Autodesk Inventor part; units mm, degrees
ref_plane "Work Plane3" through (25.4, 13.0175, 0) normal (1, 0, 0) x (0, 0, -1)
ref_plane "YZ Plane" through (0, 0, 0) normal (1, 0, 0) x (0, 1, 0)
ref_plane "XZ Plane" through (0, 0, 0) normal (0, 1, 0) x (-1, 0, 0)
sketch "Sketch1" plane through (0, 0, 0) normal (0, 1, 0) x (-1, 0, 0)
  line L0 (0, 0) -> (-50.8, 0)
  line L1 (-50.8, 0) -> (-50.8, -25.4)
  line L2 (-50.8, -25.4) -> (0, -25.4)
  line L3 (0, -25.4) -> (0, 0)
  dimension "d0" = 50.8
  dimension "d1" = 25.4
extrude "Extrusion1" add sketch "Sketch1" along normal blind 3.175
sketch "Sketch10" plane through (0, 3.175, 0) normal (0, 1, 0) x (1, 0, 0)
  line L0 (50.8, 25.4) -> (0, 25.4)
  line L1 (0, 25.4) -> (50.8, 25.4)
  line L2 (50.8, 25.4) -> (50.8, 31.75)
  line L3 (50.8, 31.75) -> (0, 31.75)
  line L4 (0, 31.75) -> (0, 25.4)
  point P0 (0, 0)
  dimension "d46" = 6.35
extrude "Extrusion7" add sketch "Sketch10" against normal blind 57.15
sketch "Sketch11" plane through (50.8, 0, 0) normal (1, 0, 0) x (0, 0, -1)
  line L0 (25.4, -53.975) -> (31.75, -53.975)
  line L1 (25.4, -53.975) -> (0, -53.975)
  line L2 (0, -53.975) -> (0, -50.8)
  line L3 (0, -50.8) -> (25.4, -50.8)
  line L4 (25.4, -50.8) -> (25.4, -53.975)
  point P0 (0, 0)
  dimension "d49" = 3.175
  dimension "d80" = 25.4
extrude "Extrusion8" add sketch "Sketch11" against normal blind 50.8
sketch "Sketch12" plane through (0, 3.175, 0) normal (0, 1, 0) x (1, 0, 0)
  line L0 (9.525, 31.75) -> (19.05, 31.75)
  line L1 (19.05, 31.75) -> (19.05, 0)
  line L2 (19.05, 0) -> (9.525, 0)
  line L3 (9.525, 0) -> (9.525, 31.75)
  line L4 (31.75, 31.75) -> (41.275, 31.75)
  line L5 (41.275, 31.75) -> (41.275, 0)
  line L6 (41.275, 0) -> (31.75, 0)
  line L7 (31.75, 0) -> (31.75, 31.75)
  line L8 (19.05, 31.75) -> (31.75, 31.75) construction
  line L9 (50.8, 25.4) -> (0, 25.4) construction
  line L10 (50.8, 31.75) -> (0, 31.75) construction
  line L11 (50.8, 0) -> (50.8, 31.75) construction
  point P0 (0, 0)
  point P1 (25.4, 31.75)
  point P2 (25.4, 31.75)
  point P3 (41.275, 15.875)
  point P4 (50.8, 15.875)
  point P5 (36.5125, 31.75)
  point P6 (25.4, 31.75)
  dimension "d52" = 12.7
  dimension "d54" = 9.525
extrude "Extrusion9" add sketch "Sketch12" along normal blind 76.2
sketch "Sketch14" plane through (0, 3.175, 0) normal (0, 1, 0) x (1, 0, 0)
  line L0 (0, 31.75) -> (0, 0)
  line L1 (0, 0) -> (50.8, 0)
  point P0 (12.7, 12.7)
  point P1 (38.1, 12.7)
  dimension "d62" = 12.7
  dimension "d63" = 12.7
  dimension "d64" = 25.4
hole "Hole3" at (12.7, 3.175, -12.7) at (38.1, 3.175, -12.7) direction (0, -1, 0) diameter 3.175 end through all
sketch "Sketch15" plane through (50.8, 3.175, -31.75) normal (0, 0, -1) x (-1, 0, 0)
  line L0 (6.35, -9.525) -> (44.45, -9.525) construction
  line L1 (44.45, -9.525) -> (44.45, -47.625) construction
  line L2 (44.45, -47.625) -> (6.35, -47.625) construction
  line L3 (6.35, -47.625) -> (6.35, -9.525) construction
  line L4 (0, 0) -> (50.8, 0) construction
  line L5 (50.8, 0) -> (50.8, -57.15) construction
  point P0 (50.8, -3.175)
  point P1 (25.4, -9.525)
  point P2 (25.4, 0)
  point P3 (44.45, -28.575)
  point P4 (50.8, -28.575)
  dimension "d72" = 38.1
hole "Hole4" at (44.45, -6.35, -31.75) at (6.35, -6.35, -31.75) at (6.35, -44.45, -31.75) at (44.45, -44.45, -31.75) direction (0, 0, 1) diameter 3.175 end through all
sketch "Sketch17" plane through (9.525, 3.175, -31.75) normal (-1, 0, 0) x (0, 0, 1)
  circle A0 centre (14.2875, 31.75) radius 14.2875
  line L0 (0, 0) -> (31.75, 0)
  line L1 (31.75, 0) -> (31.75, 76.2)
  line L2 (0, 76.2) -> (31.75, 76.2)
  line L3 (31.75, 76.2) -> (0, 76.2)
  line L4 (0, 76.2) -> (0, 33.9421)
  line L5 (0, 0) -> (0, 76.2)
  arc A1 (31.75, 42.7485) -> (0, 46.6421) centre (14.2875, 31.75) ccw
  arc A2 (0, 46.6421) -> (0, 0) centre (22.3743, 23.321) ccw
  point P0 (31.75, -3.175)
  point P1 (31.75, 30.0485)
  point P2 (0, 46.6421)
  point P3 (0, 46.6421)
  point P4 (0, 46.6421)
  dimension "d83" = 28.575
  dimension "d84" = 31.75
  dimension "d85" = 17.4625
  dimension "d98" = 6.35
extrude "Extrusion16" cut sketch "Sketch17" against normal blind 38.1 contours A0 | L4 L2 L1 A1
sketch "Sketch19" plane through (0, 0, 0) normal (0, 0, 1) x (1, 0, 0)
  line L0 (31.75, 3.175) -> (31.75, 20.0329)
  arc A0 (19.05, 15.875) -> (31.75, 15.875) centre (25.4, 14.4462) ccw
  line L1 (19.05, 3.175) -> (31.75, 3.175)
  line L2 (19.05, 3.175) -> (19.05, 45.9235)
  line L3 (31.75, 3.175) -> (31.75, 45.9235)
  point P0 (0, 0)
  point P1 (31.75, 15.875)
  dimension "d103" = 4.7625
  dimension "d104" = 12.7
  dimension "d105" = 12.7
extrude "Extrusion18" add sketch "Sketch19" against normal blind 31.75
sketch "Sketch20" plane through (19.05, 34.925, -17.4625) normal (1, 0, 0) x (0, 0, -1)
  circle A0 centre (0, 0) radius 14.2875
  circle A1 centre (0, 0) radius 15.5575
  point P0 (-17.4625, -34.925)
  dimension "d108" = 1.27
extrude "Extrusion20" add sketch "Sketch17" against normal blind 9.525 contours L5 A2 L4
extrude "Extrusion21" cut sketch "Sketch20" against normal blind 1.651
ref_plane "Work Plane3" through (25.4, 13.0175, 0) normal (1, 0, 0) x (0, 0, -1)
mirror "Mirror6" about plane through (25.4, 13.0175, 0) normal (1, 0, 0) of "Extrusion20", "Extrusion21"
sketch "Sketch21" plane through (41.275, 3.175, 0) normal (1, 0, 0) x (0, 0, -1)
  circle A0 centre (17.4625, 31.75) radius 14.2875
  arc A1 (31.75, 0) -> (31.75, 46.6421) centre (9.3757, 23.321) ccw
  arc A2 (31.75, 46.6421) -> (0, 42.7485) centre (17.4625, 31.75) ccw
  line L0 (0, 0) -> (0, 42.7485)
  line L1 (31.75, 0) -> (0, 0)
  point P0 (0, -3.175)
sketch "Sketch22" plane through (0, 3.175, 0) normal (0, 1, 0) x (1, 0, 0)
  line L0 (50.8, 0) -> (50.8, 31.75)
  line L1 (41.275, 31.75) -> (41.275, 0)
  line L2 (41.275, 0) -> (50.8, 0)
  line L3 (50.8, 0) -> (50.8, 31.75)
  line L4 (50.8, 31.75) -> (41.275, 31.75)
  point P0 (0, 0)
sketch "Sketch23" plane through (41.275, 3.175, 0) normal (1, 0, 0) x (0, 0, -1)
  circle A0 centre (17.4625, 31.75) radius 14.2875
  line L0 (14.1389, 17.8544) -> (0, 17.8544)
  line L1 (0, 0) -> (0, 42.7485)
  line L2 (14.1389, 17.8544) -> (31.75, 17.8544)
  line L3 (31.75, 0) -> (31.75, 9.8425)
  line L4 (31.75, 17.8544) -> (31.75, 0)
  point P0 (0, -3.175)
sketch "Sketch24" plane through (0, 0, 0) normal (0, 0, 1) x (1, 0, 0)
  line L0 (50.8, 0) -> (50.8, 3.175)
  line L1 (50.8, 3.175) -> (41.275, 19.9074)
  line L2 (41.275, 49.8171) -> (41.275, 3.175)
  line L3 (41.275, 21.0294) -> (41.275, 3.175)
  line L4 (41.275, 3.175) -> (50.8, 3.175)
  line L5 (41.275, 3.175) -> (50.8, 3.175)
  point P0 (0, 0)
extrude "Extrusion22" add sketch "Sketch24" against normal blind 31.75
mirror "Mirror7" about plane through (25.4, 13.0175, 0) normal (1, 0, 0) of "Extrusion22"
properties part number "Intake - Mount"
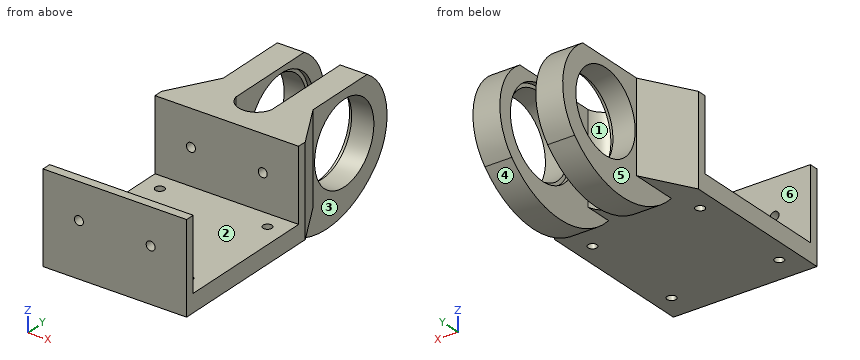
Design review of the part built by this model. Coordinates are the model's own, in mm. Face numbers are marked on the shaded views. A direction names the side the tool comes from. Give positions to 0.01 mm unless a question says otherwise; leave off trailing zeros. Write each loop counter-clockwise with the first axis right and the second up, starting at its lowest first coordinate (ties: lowest second). Pieces come first, ordered by that corner, then holes. Notation, with made-up numbers: M 69,17 L 105,17 A18 ccw 105,22 Z; hole C -28.5,-11.5 d10. An arc over 180 degrees is marked long. Return JSON: item names as keys, results as strings. Group by question number.
Item 1: The part is to be moulded in two halves that separate along X. For the marked faces 1, 2 and 3, say which applies: pulls with the +X half, pulls with the -X half, needs draft (parallel to the pull), parting line crosses it, or undercut.
Item 2: Tool access review of the marked faces 4, 5 and 6: name each direction out of +Z, -Z, +X, -X, +Y, -Y from which nothing blocks a thin tool from reaching the whole face with its end or side.
Item 3: Take a section at A-A (x = 12.7). Count the separate pieces of the cut face and the enclosed holes in it, plus the area to 3 significant figures.
Item 4: Take a section at B-B (y = -44.45). Give the boundary of the cut face in (x, z), plus the area to 3 significant figures.
Item 5: Clearance check with flat-ended pins moving along their axes: pin 1 Ø6 at (x, z) = (27, -21.5) entering from +Y; pin 2 Ø4 at (x, y) = (44.45, -6.35) entering from +Z; pin 3 Ø3.5 at (x, z) = (12.7, -12.7) entering from -Y (3 decimals); pin 4 Ø3 at (x, z) = (38.1, -12.7) entering from +Y. State where each tip first meets the part, or that it passes through.
Item 6: Wall thickness on line 1 along Y through (x, z) = (17, -24) (3 decimals); line 2 along X through (y, z) = (31, -37) (3 decimals); line 3 along Y through (x, z) = (10.5, -11) (3 decimals): over which ranges is each line inside the solid? List them lowest first.
Return value:
{
 "1": {"face 1": "undercut", "face 2": "needs draft", "face 3": "pulls with the +X half"},
 "2": {"face 4": "-Z, +X, -X", "face 5": "-Z, -X, +Y", "face 6": "+Z, +X, -X"},
 "3": {"separate pieces": "2", "enclosed holes": "1", "area": "1,770 mm2"},
 "4": {"outline": "M 0,-31.75 L 4.76,-31.75 L 4.76,-25.4 L 0,-25.4 Z; M 7.94,-31.75 L 42.86,-31.75 L 42.86,-25.4 L 7.94,-25.4 Z; M 46.04,-31.75 L 50.8,-31.75 L 50.8,-25.4 L 46.04,-25.4 Z", "area": "282 mm2"},
 "5": {"pin 1": "stops at y = 9.84", "pin 2": "stops at z = -25.4", "pin 3": "stops at y = -53.975", "pin 4": "stops at y = 55.3"},
 "6": {"line 1": "y = -53.975 to -50.8, 0 to 22.221, 47.629 to 54.5", "line 2": "x = 9.525 to 19.05, 31.75 to 41.275", "line 3": "y = -53.975 to -50.8, 0 to 22.183, 47.667 to 54.525"}
}
